Can you work these out from the model? Positions are in its coordinate system, mm. Round coordinates to 2 decimals unless told otherwise and drop trailing zeros. One line per question, with ' | ' between items.
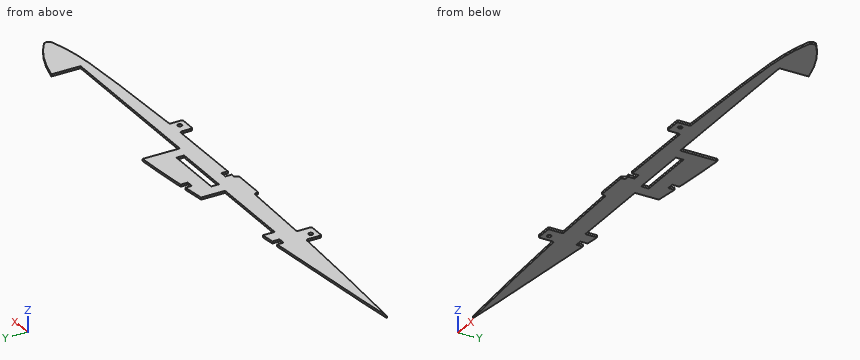
```python
from build123d import *

# Parameters (mm, degrees)
BOSS_EXTRUDE1_DEPTH = 3.175
FILLET1_R           = 6.35
SKETCH6_W           = 88.9
SKETCH6_H           = 11.43
CUT_EXTRUDE3_DEPTH  = 5.08
SKETCH3_W           = 25.4
SKETCH3_H           = 3.175
BOSS_EXTRUDE2_DEPTH = 31.75
SKETCH3_3_W         = 50.8
SKETCH3_3_H         = 3.175
BOSS_EXTRUDE3_DEPTH = 19.05
FILLET2_R           = 2.54
CUT_EXTRUDE2_DEPTH  = 12.7
CUT_EXTRUDE4_DEPTH  = 5.08
SKETCH8_R           = 3.175
CUT_EXTRUDE5_DEPTH  = 504.378680986
CAVITY1_START       = 46.415619464
CAVITY1_OUTLINE_W   = 10.16
CAVITY1_OUTLINE_H   = 3.175
CAVITY1_DEPTH       = 10.772258138
CAVITY1_START_2     = 20.382459347
CAVITY1_2_OUTLINE_W = 10.16
CAVITY1_2_OUTLINE_H = 3.175
CAVITY1_2_DEPTH     = 10.743999494
CAVITY1_START_3     = -13.279272859
CAVITY1_3_OUTLINE_W = 10.16
CAVITY1_3_OUTLINE_H = 3.175
CAVITY1_3_DEPTH     = 9.525


# Read off the part's stored shape, not the designer's step: Cavity1
with BuildPart() as part:
    # Sketch1 → Boss-Extrude1 (new body)
    with BuildSketch(Plane.XY):
        with BuildLine():
            add(Edge.make_bspline(
                [(-353.097115344, 3.76640622), (-263.60988857, 15.489732087), (-103.405625954, 27.702523148), (139.625383809, 69.731889132), (320.600909148, 70.897971745), (447.029350736, 49.156772515), (484.461992977, 32.39779841), (505.225432444, 13.29140622)],
                knots=[0, 0, 0, 0, 0.308401543, 0.542913332, 0.850169973, 0.887176211, 1, 1, 1, 1], degree=3))
            add(Edge.make_bspline(
                [(-353.097115344, 3.76640622), (-171.204173065, -8.622681299), (70.681231732, -17.726989966), (367.634485174, -8.589262826), (467.934967897, -1.634661846), (505.225432444, 13.29140622)],
                knots=[0, 0, 0, 0, 0.625313044, 0.861778666, 1, 1, 1, 1], degree=3))
        make_face()
    extrude(amount=BOSS_EXTRUDE1_DEPTH)

    # Fillet1
    fillet1_edges = [part.edges().sort_by_distance(p)[0] for p in [
        (505.225432444, 13.29140622, 1.5875),
    ]]
    fillet(fillet1_edges, radius=FILLET1_R)

    # Sketch6 → Cut-Extrude3 (cut)
    with BuildSketch(Plane.XY):
        with Locations((104.102884656, 19.812)):
            Rectangle(SKETCH6_W, SKETCH6_H)
    extrude(amount=CUT_EXTRUDE3_DEPTH, mode=Mode.SUBTRACT)

    # Sketch3 → Boss-Extrude2 (add)
    with BuildSketch(Plane(origin=(0, 0, 0), x_dir=(1, 0, 0), z_dir=(0, 1, 0))):
        with Locations((-111.797115344, -1.5875)):
            Rectangle(SKETCH3_W, SKETCH3_H)
        with Locations((218.402884656, -1.5875)):
            Rectangle(SKETCH3_W, SKETCH3_H)
    extrude(amount=-BOSS_EXTRUDE2_DEPTH)

    # Sketch3<3> → Boss-Extrude3 (add)
    with BuildSketch(Plane(origin=(0, 0, 0), x_dir=(1, 0, 0), z_dir=(0, 1, 0))):
        with Locations((40.53772502, -1.5875)):
            Rectangle(SKETCH3_3_W, SKETCH3_3_H)
    extrude(amount=-BOSS_EXTRUDE3_DEPTH)

    # Fillet2
    fillet2_edges = [part.edges().sort_by_distance(p)[0] for p in [
        (-124.497115344, -8.618440951, 1.5875),
        (-99.097115344, -9.553641032, 1.5875),
        (205.702884656, -12.629236372, 1.5875),
        (231.102884656, -12.164410009, 1.5875),
        (15.13772502, -12.521395898, 1.5875),
        (65.93772502, -13.158984983, 1.5875),
        (-124.497115344, -31.75, 1.5875),
        (-99.097115344, -31.75, 1.5875),
        (15.13772502, -19.05, 1.5875),
        (65.93772502, -19.05, 1.5875),
        (205.702884656, -31.75, 1.5875),
        (231.102884656, -31.75, 1.5875),
    ]]
    fillet(fillet2_edges, radius=FILLET2_R)

    # Sketch5 → Cut-Extrude2 (cut, symmetric)
    with BuildSketch(Plane.XY):
        with BuildLine():
            Line((167.602884656, 9.525), (421.602884656, 9.525))
            Line((421.602884656, 9.525), (421.602884656, 53.128136288))
            add(Edge.make_bspline(
                [(167.602884656, 65.051503813), (244.722722107, 70.03272949), (333.181087562, 68.488590043), (412.953469478, 55.01226242), (421.602884656, 53.128136288)],
                knots=[0.603089435, 0.603089435, 0.603089435, 0.603089435, 0.862957728, 0.895261032, 0.895261032, 0.895261032, 0.895261032], degree=3))
            Line((167.602884656, 65.051503813), (167.602884656, 9.525))
        make_face()
    extrude(amount=CUT_EXTRUDE2_DEPTH, both=True, mode=Mode.SUBTRACT)

    # Sketch7 → Cut-Extrude4 (cut)
    with BuildSketch(Plane.XY):
        with BuildLine():
            Line((40.602884656, 51.591569772), (40.602884656, 15.875))
            Line((40.602884656, 15.875), (-86.397115344, 15.875))
            Line((-86.397115344, 15.875), (-86.397115344, 33.671872302))
            add(Edge.make_bspline(
                [(-86.397115344, 33.671872302), (-85.336997309, 33.80875443), (-42.923565209, 39.312219047), (-0.873657075, 45.877823306), (40.602884656, 51.591569772)],
                knots=[0.304745552, 0.304745552, 0.304745552, 0.304745552, 0.308401543, 0.451045815, 0.451045815, 0.451045815, 0.451045815], degree=3))
        make_face()
    extrude(amount=CUT_EXTRUDE4_DEPTH, mode=Mode.SUBTRACT)

    # Sketch8 → Cut-Extrude5 (cut, through all)
    with BuildSketch(Plane.XY):
        with Locations((220.942884656, -21.59)):
            Circle(SKETCH8_R)
        with Locations((-114.337115344, -21.59)):
            Circle(SKETCH8_R)
    extrude(amount=CUT_EXTRUDE5_DEPTH, mode=Mode.SUBTRACT)

    # Cavity1 outline → Cavity1 (cut)
    with BuildSketch(Plane(origin=(0, 0, 0), x_dir=(1, 0, 0), z_dir=(0, 1, 0)).offset(CAVITY1_START)):
        with Locations((78.637724966, -1.5875)):
            Rectangle(CAVITY1_OUTLINE_W, CAVITY1_OUTLINE_H)
    extrude(amount=CAVITY1_DEPTH, mode=Mode.SUBTRACT)

    # Cavity1 2 outline → Cavity1 2 (cut)
    with BuildSketch(Plane(origin=(0, 0, 0), x_dir=(1, 0, 0), z_dir=(0, 1, 0)).offset(CAVITY1_START_2)):
        with Locations((-111.797115344, -1.5875)):
            Rectangle(CAVITY1_2_OUTLINE_W, CAVITY1_2_OUTLINE_H)
    extrude(amount=CAVITY1_2_DEPTH, mode=Mode.SUBTRACT)

    # Cavity1 3 outline → Cavity1 3 (cut)
    with BuildSketch(Plane(origin=(0, 0, 0), x_dir=(1, 0, 0), z_dir=(0, 1, 0)).offset(CAVITY1_START_3)):
        with Locations((78.637724966, -1.5875)):
            Rectangle(CAVITY1_3_OUTLINE_W, CAVITY1_3_OUTLINE_H)
    extrude(amount=CAVITY1_3_DEPTH, mode=Mode.SUBTRACT)


solid = part.part
```
(1) Will these pins go through, and if not, where does the flat tip stop? pin 1 Ø1 at (x, z) = (79, 2.5) entering from +Y; pin 2 Ø1 at (y, z) = (20, 1) entering from +X; pin 3 Ø1.6 at (x, z) = (308.5, 1.5) entering from +Y (3 decimals).
Final values:
pin 1: y = 46.42 | pin 2: x = 497.69 | pin 3: y = 9.525
(2) Please list where these lines run through material, in increasing order: probe 1 along X at (y, z) = (-21.59, 1.1); probe 2 along X at (y, z) = (-22.5, 2.25); probe 3 along Y at (x, z) = (216.5, 1.8) (3 decimals). Write a range as [from, to].
Final values:
probe 1: [-124.5, -117.51], [-111.16, -99.1], [205.7, 217.77], [224.12, 231.1] | probe 2: [-124.5, -117.38], [-111.3, -99.1], [205.7, 217.9], [223.98, 231.1] | probe 3: [-31.75, 9.525]
(3) If we section it at A-A on z = 2.45: State how many separate pieces and enclosed holes the cut face has, plus the area to 3 significant figures.
Final values:
separate pieces: 1 | enclosed holes: 3 | area: 26,600 mm^2
